from build123d import *

# Parameters (mm, degrees)
BOSS_EXTRU_2_DEPTH      = 18
ESQUISSE1_W             = 100
ESQUISSE1_H             = 30
ENL_V_MAT_EXTRU_1_DEPTH = 19
CONG_1_R                = 7


with BuildPart() as part:
    # Esquisse2 → Boss.-Extru.2 (new body)
    with BuildSketch(Plane.XY):
        Polygon((0, 0), (350, 0), (350, -250), (50, -250), (50, -100), (0, -100), align=None)
    extrude(amount=BOSS_EXTRU_2_DEPTH)

    # Esquisse1 → Enlèv. mat.-Extru.1 (cut, through all)
    with BuildSketch(Plane.XY):
        with BuildLine():
            Line((106.489567957, -120.054539114), (166.945460886, -180.510432043))
            ThreePointArc((166.945460886, -180.510432043), (167.433604863, -180.857617354), (168.008646739, -181.025394064))
            ThreePointArc((168.008646739, -181.025394064), (172.426406871, -185.991378029), (168.008646739, -190.957361993))
            ThreePointArc((168.008646739, -190.957361993), (167.433604863, -191.125138703), (166.945460886, -191.472324014))
            Line((166.945460886, -191.472324014), (164.472324014, -193.945460886))
            ThreePointArc((164.472324014, -193.945460886), (164.125138703, -194.433604863), (163.957361993, -195.008646739))
            ThreePointArc((163.957361993, -195.008646739), (158.991378029, -199.426406871), (154.025394064, -195.008646739))
            ThreePointArc((154.025394064, -195.008646739), (153.857617354, -194.433604863), (153.510432043, -193.945460886))
            Line((153.510432043, -193.945460886), (93.054539114, -133.489567957))
            ThreePointArc((93.054539114, -133.489567957), (92.566395137, -133.142382646), (91.991353261, -132.974605936))
            ThreePointArc((91.991353261, -132.974605936), (87.573593129, -128.008621971), (91.991353261, -123.042638007))
            ThreePointArc((91.991353261, -123.042638007), (92.566395137, -122.874861297), (93.054539114, -122.527675986))
            Line((93.054539114, -122.527675986), (95.527675986, -120.054539114))
            ThreePointArc((95.527675986, -120.054539114), (95.874861297, -119.566395137), (96.042638007, -118.991353261))
            ThreePointArc((96.042638007, -118.991353261), (101.008621971, -114.573593129), (105.974605936, -118.991353261))
            ThreePointArc((105.974605936, -118.991353261), (106.142382646, -119.566395137), (106.489567957, -120.054539114))
        make_face()
        with BuildLine():
            Line((50, -100), (30, -100))
            Line((30, -100), (30.424047381, -57.1712145))
            ThreePointArc((30.424047381, -57.1712145), (30.332595572, -56.586679793), (30.056564564, -56.06337191))
            ThreePointArc((30.056564564, -56.06337191), (30.532330845, -49.467962139), (37.135309084, -49.11234721))
            ThreePointArc((37.135309084, -49.11234721), (37.660561143, -49.400327171), (38.251228148, -49.5))
            Line((38.251228148, -49.5), (41.748771852, -49.5))
            ThreePointArc((41.748771852, -49.5), (42.339438857, -49.400327171), (42.864690916, -49.11234721))
            ThreePointArc((42.864690916, -49.11234721), (49.467669155, -49.467962139), (49.943435436, -56.06337191))
            ThreePointArc((49.943435436, -56.06337191), (49.667404428, -56.586679793), (49.575952619, -57.1712145))
            Line((49.575952619, -57.1712145), (50, -100))
        make_face()
        with Locations((200, -45)):
            Rectangle(ESQUISSE1_W, ESQUISSE1_H)
        with BuildLine():
            Line((304.472324014, -120.054539114), (306.945460886, -122.527675986))
            ThreePointArc((306.945460886, -122.527675986), (307.433604863, -122.874861297), (308.008646739, -123.042638007))
            ThreePointArc((308.008646739, -123.042638007), (312.426406871, -128.008621971), (308.008646739, -132.974605936))
            ThreePointArc((308.008646739, -132.974605936), (307.433604863, -133.142382646), (306.945460886, -133.489567957))
            Line((306.945460886, -133.489567957), (246.489567957, -193.945460886))
            ThreePointArc((246.489567957, -193.945460886), (246.142382646, -194.433604863), (245.974605936, -195.008646739))
            ThreePointArc((245.974605936, -195.008646739), (241.008621971, -199.426406871), (236.042638007, -195.008646739))
            ThreePointArc((236.042638007, -195.008646739), (235.874861297, -194.433604863), (235.527675986, -193.945460886))
            Line((235.527675986, -193.945460886), (233.054539114, -191.472324014))
            ThreePointArc((233.054539114, -191.472324014), (232.566395137, -191.125138703), (231.991353261, -190.957361993))
            ThreePointArc((231.991353261, -190.957361993), (227.573593129, -185.991378029), (231.991353261, -181.025394064))
            ThreePointArc((231.991353261, -181.025394064), (232.566395137, -180.857617354), (233.054539114, -180.510432043))
            Line((233.054539114, -180.510432043), (293.510432043, -120.054539114))
            ThreePointArc((293.510432043, -120.054539114), (293.857617354, -119.566395137), (294.025394064, -118.991353261))
            ThreePointArc((294.025394064, -118.991353261), (298.991378029, -114.573593129), (303.957361993, -118.991353261))
            ThreePointArc((303.957361993, -118.991353261), (304.125138703, -119.566395137), (304.472324014, -120.054539114))
        make_face()
    extrude(amount=ENL_V_MAT_EXTRU_1_DEPTH, mode=Mode.SUBTRACT)

    # Congé1
    cong_1_edges = [part.edges().sort_by_distance(p)[0] for p in [
        (0, 0, 9),
        (350, 0, 9),
        (350, -250, 9),
        (50, -250, 9),
        (0, -100, 9),
        (150, -30, 9),
        (150, -60, 9),
        (250, -60, 9),
        (250, -30, 9),
        (30, -100, 9),
    ]]
    fillet(cong_1_edges, radius=CONG_1_R)


solid = part.part
Check sheet for the modelled part. Datum: model origin and axes. Units: mm. A direction names the side the tool comes from. Round coordinates to 2 decimals unless told otherwise and drop trailing zeros. Loops run counter-clockwise (first coordinate to the right, second up) from the corner with the lowest first, then second, coordinate; pieces in that order, holes last. Notation, with made-up numbers: (71, 78) - (88, 78) arc R20 ccw to (88, 82) - close; hole circle Ø1 at (-0.75, 39). An arc over 180 degrees is marked (long way). Answer as CSV lines item,"result". Start each with the question number.
Item 1: Section check A-A (x = 215). Record the boundary of the cut face in (y, z).
Item 2: Release check for a two-part mould opening along Y. For faces 1 (the flat face through (0, -51, 9)), 2 (the flat face through (123.706, -164.141, 8.874)), 3 (the cylindrical face through (347.9, -2, 9.1)) record: +Y half, -Y half, draft (parallel to the pull), parting line (faces both ways), or undercut.
Item 3: Section check C-C (y = -73.5). Record the boundary of the cut face in (x, z), and give its area (3 significant figures).
Item 4: Set-up check for faces 4 (the flat face through (177, -123, 0)), 5 (the cylindrical face through (247.9, -32, 9.1)), 6 (the flat face through (50, -173, 9)): record each of +Z, -Z, +X, -X, +Y, -Y from which the full face is reachable in a straight line by a thin tool's end or side.
Item 5: Scan lines: line 1 (X direction, y = -65, z = 8); line 2 (Y direction, x = 213.5, z = 16.5); line 3 (X direction, y = -157, z = 9.25). Record each from-to range of solid material in increasing order. Write a range as [from, to].
Item 6: Section check D-D (z = 13.5). Count the separate pieces of the cut face and the enclosed holes in it, and give its area (3 significant figures).
Item 7: Depth check by flat-ended pin: P1, Ø8, axis at x = 11.5, z = 10, coming from the -Y side; P2, Ø3, axis at x = 40.5, z = 13.5, coming from the -Y side. Enter the tip coordinate at first touch or a pass-through.
Item 8: Section check B-B (y = -159). Record the boundary of the cut face in (x, z), and give its area (3 significant figures).
Report:
1,outline,"(-250, 0) - (-60, 0) - (-60, 18) - (-250, 18) - close; (-30, 0) - (0, 0) - (0, 18) - (-30, 18) - close"
2,face 1,"draft"
2,face 2,"undercut"
2,face 3,"+Y half"
3,outline,"(0, 0) - (30.26, 0) - (30.26, 18) - (0, 18) - close; (49.74, 0) - (350, 0) - (350, 18) - (49.74, 18) - close"
3,area,"5,950 mm2"
4,face 4,"-Z, +X, -X, +Y, -Y"
4,face 5,"+Z, -Z"
4,face 6,"+Z, -Z, -X, -Y"
5,line 1,"x = [0, 30.35], [49.65, 350]"
5,line 2,"y = [-250, -60], [-30, 0]"
5,line 3,"x = [50, 116.56], [143.44, 256.56], [283.44, 350]"
6,separate pieces,"1"
6,enclosed holes,"3"
6,area,"72,000 mm2"
7,P1,"stops at y = -100"
7,P2,"stops at y = -49.5"
8,outline,"(50, 0) - (118.56, 0) - (118.56, 18) - (50, 18) - close; (145.44, 0) - (254.56, 0) - (254.56, 18) - (145.44, 18) - close; (281.44, 0) - (350, 0) - (350, 18) - (281.44, 18) - close"
8,area,"4,430 mm2"
